from build123d import *

# Parameters (mm, degrees)
BOSS_EXTRUDE1_DEPTH = 45
SKETCH2_R           = 11
CUT_EXTRUDE1_DEPTH  = 5
SKETCH3_R           = 1.5
CUT_EXTRUDE2_DEPTH  = 5
SKETCH4_R           = 2
CUT_EXTRUDE3_DEPTH  = 5
SKETCH5_R           = 2
CUT_EXTRUDE4_DEPTH  = 5


with BuildPart() as part:
    # Sketch1 → Boss-Extrude1 (new body)
    with BuildSketch(Plane.XY):
        Polygon((0, 50), (0, 0), (-50, 0), (-50, 5), (-5, 5), (-5, 50), align=None)
    extrude(amount=BOSS_EXTRUDE1_DEPTH)

    # Sketch2 → Cut-Extrude1 (cut)
    with BuildSketch(Plane(origin=(0, 0, 0), x_dir=(0, 0, -1), z_dir=(1, 0, 0))):
        with Locations((-22.5, 22)):
            Circle(SKETCH2_R)
    extrude(amount=-CUT_EXTRUDE1_DEPTH, mode=Mode.SUBTRACT)

    # Sketch3 → Cut-Extrude2 (cut)
    with BuildSketch(Plane(origin=(0, 0, 0), x_dir=(0, 0, -1), z_dir=(1, 0, 0))):
        with Locations((-22.5, 35.5)):
            Circle(SKETCH3_R)
        with Locations((-9, 22)):
            Circle(SKETCH3_R)
        with Locations((-22.5, 8.5)):
            Circle(SKETCH3_R)
        with Locations((-36, 22)):
            Circle(SKETCH3_R)
    extrude(amount=-CUT_EXTRUDE2_DEPTH, mode=Mode.SUBTRACT)

    # Sketch4 → Cut-Extrude3 (cut)
    with BuildSketch(Plane(origin=(0, 5, 0), x_dir=(1, 0, 0), z_dir=(0, 1, 0))):
        with Locations(Location((-27.5, -5.290295093, 0), (0, 0, 270))):
            Circle(SKETCH4_R)
        with Locations(Location((-15.330900958, -10.330900958, 0), (0, 0, 270))):
            Circle(SKETCH4_R)
        with Locations(Location((-10.290295093, -22.5, 0), (0, 0, 270))):
            Circle(SKETCH4_R)
        with Locations(Location((-15.330900958, -34.669099042, 0), (0, 0, 270))):
            Circle(SKETCH4_R)
        with Locations(Location((-27.5, -39.709704907, 0), (0, 0, 270))):
            Circle(SKETCH4_R)
        with Locations(Location((-39.669099042, -34.669099042, 0), (0, 0, 270))):
            Circle(SKETCH4_R)
        with Locations(Location((-44.709704907, -22.5, 0), (0, 0, 270))):
            Circle(SKETCH4_R)
        with Locations(Location((-39.669099042, -10.330900958, 0), (0, 0, 270))):
            Circle(SKETCH4_R)
    extrude(amount=-CUT_EXTRUDE3_DEPTH, mode=Mode.SUBTRACT)

    # Sketch5 → Cut-Extrude4 (cut)
    with BuildSketch(Plane(origin=(0, 0, 0), x_dir=(0, 0, -1), z_dir=(1, 0, 0))):
        with Locations((-37, 43.708447977)):
            Circle(SKETCH5_R)
        with Locations(Location((-8, 43.708447977, 0), (0, 0, 180))):
            Circle(SKETCH5_R)
    extrude(amount=-CUT_EXTRUDE4_DEPTH, mode=Mode.SUBTRACT)


solid = part.part
Geometry check sheet. Reference: the model listing, model coordinates, mm. A direction names the side the tool comes from. Give positions to 0.01 mm unless a question says otherwise; leave off trailing zeros. Write each loop counter-clockwise with the first axis right and the second up, starting at its lowest first coordinate (ties: lowest second). Pieces come first, ordered by that corner, then holes.
1) Release check for a two-part mould opening along X. For faces 3 (the face through (-8.939, 2.535, 21.026)), 4 (the face through (-50, 2, 22)), 5 (the face through (-2.5, 7.6, 23.7)) record: released by +X, released by -X, zero draft, split by the parting line, or undercut.
Values follow:
face 3: undercut
face 4: released by -X
face 5: zero draft
2) Cross-section at B-B (y = 35.5). Record the boundary of the cut face in (x, z).
Values follow:
outline: (-5, 0) - (0, 0) - (0, 21) - (-5, 21) - close; (-5, 24) - (0, 24) - (0, 45) - (-5, 45) - close
3) Cross-section at C-C (x = -9.5). Record the boundary of the cut face in (y, z), plus the area to 3 significant figures.
Values follow:
outline: (0, 0) - (5, 0) - (5, 20.66) - (0, 20.66) - close; (0, 24.34) - (5, 24.34) - (5, 45) - (0, 45) - close
area: 207 mm2
4) Cross-section at A-A (x = -27.5). Record the boundary of the cut face in (y, z).
Values follow:
outline: (0, 0) - (5, 0) - (5, 3.29) - (0, 3.29) - close; (0, 7.29) - (5, 7.29) - (5, 37.71) - (0, 37.71) - close; (0, 41.71) - (5, 41.71) - (5, 45) - (0, 45) - close
5) Go/stop test with flat-tipped pins: pin 1 Ø3.5 at (x, z) = (-15.33, 34.67) entering from -Y; pin 2 Ø4 at (y, z) = (35.5, 22.5) entering from -X; pin 3 Ø6.5 at (x, z) = (-39.67, 34.67) entering from +Y. Record where each tip stops, or that it passes through.
Values follow:
pin 1: passes through
pin 2: stops at x = -5
pin 3: stops at y = 5
6) Set-up check for faces 1 (the face through (-5, 32, 17)), 2 (the face through (-40.435, 2.535, 36.517)): record each of +Z, -Z, +X, -X, +Y, -Y from which the full face is reachable in a straight line by a thin tool's end or side.
Values follow:
face 1: +Z, -Z, -X, +Y
face 2: +Y, -Y
7) Thickness scan on line 1 (Y direction, x = -3.5, z = 9.5); line 2 (X direction, y = 43, z = 26); line 3 (Y direction, x = -1, z = 8). Record the ranges inside material, lowest first.
Values follow:
line 1: y = 0 to 20.59, 23.41 to 42.39, 45.03 to 50
line 2: x = -5 to 0
line 3: y = 0 to 20.88, 23.12 to 41.71, 45.71 to 50
8) Cross-section at D-D (y = 22). Record the boundary of the cut face in (x, z), plus the area to 3 significant figures.
Values follow:
outline: (-5, 0) - (0, 0) - (0, 7.5) - (-5, 7.5) - close; (-5, 10.5) - (0, 10.5) - (0, 11.5) - (-5, 11.5) - close; (-5, 33.5) - (0, 33.5) - (0, 34.5) - (-5, 34.5) - close; (-5, 37.5) - (0, 37.5) - (0, 45) - (-5, 45) - close
area: 85.0 mm2
